Autodesk Inventor part; units mm, degrees
ref_plane "YZ Plane" through (0, 0, 0) normal (1, 0, 0) x (0, 1, 0)
ref_plane "XZ Plane" through (0, 0, 0) normal (0, 1, 0) x (-1, 0, 0)
ref_plane "XY Plane" through (0, 0, 0) normal (0, 0, 1) x (1, 0, 0)
sketch "Sketch1" plane through (0, 0, 0) normal (0, 1, 0) x (-1, 0, 0)
  line L0 (1.7985, -1.0383) -> (0, -2.0767)
  line L1 (0, -2.0767) -> (-1.7985, -1.0383)
  line L2 (-1.7985, -1.0383) -> (-1.7985, 1.0383)
  line L3 (-1.7985, 1.0383) -> (0, 2.0767)
  line L4 (0, 2.0767) -> (1.7985, 1.0383)
  line L5 (1.7985, 1.0383) -> (1.7985, -1.0383)
  point P0 (0, 0)
  point P1 (0, 0)
  point P2 (0, 0)
extrude "Extrusion1" add sketch "Sketch1" along normal blind 4
sketch "Sketch2" plane through (0, 4, 0) normal (0, 1, 0) x (1, 0, 0)
  circle A0 centre (0, 0) radius 1.5
  dimension "d3" = 3
extrude "Extrusion2" add sketch "Sketch2" along normal blind 3
thread "Thread1"
sketch "Sketch3" plane through (0, 0, 0) normal (0, -1, 0) x (1, 0, 0)
  circle A0 centre (0, 0) radius 1.5
  dimension "d8" = 3
extrude "Extrusion3" cut sketch "Sketch3" against normal blind 3
thread "Thread2"
properties part number "Standoff"
Here's how the part is built. I have some questions about the finished solid (model axes, mm). A direction names the side the tool comes from. Coordinates: 2 decimals unless noted, no trailing zeros. Write each loop counter-clockwise with the first axis right and the second up, starting at its lowest first coordinate (ties: lowest second). Pieces come first, ordered by that corner, then holes.
Item 1: I want a section at C-C on z = 1.15. Write out the boundary of the cut face in (x, y).
Item 2: I want a section at A-A on y = 1. Write out the boundary of the cut face in (x, z).
Item 3: If I drill on line 1 (Y direction, x = -1.45, z = -0.75); line 2 (X direction, y = 5, z = -0.05); line 3 (Y direction, x = 0, z = 1), over which ranges is the centre line in solid material (lowest first)?
Item 4: If we mould it in two halves opening along Z, with no side actions, what happens to faces 4 (the flat face through (0.887, 1.972, -1.565)), 5 (the cylindrical face through (-1.5, 1.48, 0.07)), 6 (the flat face through (-1.798, 2, 0))? For each: +Z half, -Z half, draft (parallel to the pull), parting line (faces both ways), or undercut.
Item 5: I want a section at B-B on y = 3.75. Write out the boundary of the cut face in (x, z), and give its area (3 significant figures).
Item 6: On a 3-axis mill with a long thin cutter (end or side, diameter ignored), from which of +Z, -Z, +X, -X, +Y, -Y can I reach the whole of each face in a straight line? I mean faces 1 (the cylindrical face through (-1.5, 5.48, 0.07)), 2 (the flat face through (0, 3, 0)), 3 (the flat face through (-0.887, 1.972, 1.565)). Say none if no direction works.
Item 7: Will these pins go through, and if not, where does the flat tip stop? pin 1 (0.9 mm diameter, centred on x = -0.5, z = -0.5, fed in from -Y); pin 2 (1.5 mm diameter, centred on x = 1, y = 5, fed in from +Z); pin 3 (1.5 mm diameter, centred on x = 0, y = 6, fed in from -Z).
Item 8: I want a section at D-D on x = 0.4. Write out the boundary of the cut face in (y, z).
Findings below:
1. outline: (-1.61, 0) - (-0.96, 0) - (-0.96, 3) - (0.96, 3) - (0.96, 0) - (1.61, 0) - (1.61, 4) - (0.96, 4) - (0.96, 7) - (-0.96, 7) - (-0.96, 4) - (-1.61, 4) - close
2. outline: (-1.8, -1.04) - (0, -2.08) - (1.8, -1.04) - (1.8, 1.04) - (0, 2.08) - (-1.8, 1.04) - close; hole circle Ø3 at (0, 0)
3. line 1: y = 0 to 4
3. line 2: x = -1.5 to 1.5
3. line 3: y = 3 to 7
4. face 4: -Z half
4. face 5: undercut
4. face 6: draft
5. outline: (-1.8, -1.04) - (0, -2.08) - (1.8, -1.04) - (1.8, 1.04) - (0, 2.08) - (-1.8, 1.04) - close
5. area: 11.2 mm2
6. face 1: +Y
6. face 2: -Y
6. face 3: +Z, -X, +Y, -Y
7. pin 1: stops at y = 3
7. pin 2: stops at z = 1.48
7. pin 3: stops at z = -1.5
8. outline: (0, -1.85) - (4, -1.85) - (4, -1.45) - (7, -1.45) - (7, 1.45) - (4, 1.45) - (4, 1.85) - (0, 1.85) - (0, 1.45) - (3, 1.45) - (3, -1.45) - (0, -1.45) - close
